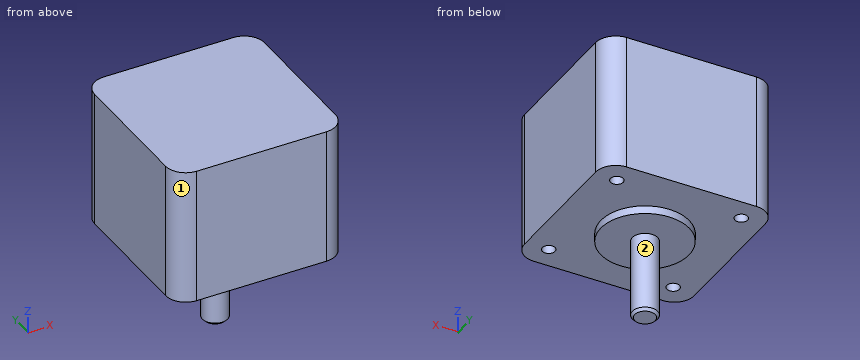
from build123d import *

# Parameters (mm, degrees)
SKETCH1_R           = 1.5875
BOSS_EXTRUDE1_DEPTH = 32
BOSS_EXTRUDE2_DEPTH = 2
SKETCH3_R           = 11
BOSS_EXTRUDE3_DEPTH = 2
SKETCH4_R           = 3.175
BOSS_EXTRUDE4_DEPTH = 20
CHAMFER1_SIZE       = 0.635


with BuildPart() as part:
    # Sketch1 → Boss-Extrude1 (new body)
    with BuildSketch(Plane.XY):
        with BuildLine():
            Line((-16.15, -21.15), (16.15, -21.15))
            ThreePointArc((16.15, -21.15), (19.685533906, -19.685533906), (21.15, -16.15))
            Line((21.15, -16.15), (21.15, 16.15))
            ThreePointArc((21.15, 16.15), (19.685533906, 19.685533906), (16.15, 21.15))
            Line((16.15, 21.15), (-16.15, 21.15))
            ThreePointArc((-16.15, 21.15), (-19.685533906, 19.685533906), (-21.15, 16.15))
            Line((-21.15, 16.15), (-21.15, -16.15))
            ThreePointArc((-21.15, -16.15), (-19.685533906, -19.685533906), (-16.15, -21.15))
        make_face()
        with Locations((15.5, 15.5)):
            Circle(SKETCH1_R, mode=Mode.SUBTRACT)
        with Locations((-15.5, 15.5)):
            Circle(SKETCH1_R, mode=Mode.SUBTRACT)
        with Locations((15.5, -15.5)):
            Circle(SKETCH1_R, mode=Mode.SUBTRACT)
        with Locations((-15.5, -15.5)):
            Circle(SKETCH1_R, mode=Mode.SUBTRACT)
    extrude(amount=BOSS_EXTRUDE1_DEPTH)

    # Sketch2 → Boss-Extrude2 (add)
    with BuildSketch(Plane.XY.offset(32)):
        with BuildLine():
            Line((-16.15, -21.15), (16.15, -21.15))
            ThreePointArc((16.15, -21.15), (19.685533906, -19.685533906), (21.15, -16.15))
            Line((21.15, -16.15), (21.15, 16.15))
            ThreePointArc((21.15, 16.15), (19.685533906, 19.685533906), (16.15, 21.15))
            Line((16.15, 21.15), (-16.15, 21.15))
            ThreePointArc((-16.15, 21.15), (-19.685533906, 19.685533906), (-21.15, 16.15))
            Line((-21.15, 16.15), (-21.15, -16.15))
            ThreePointArc((-21.15, -16.15), (-19.685533906, -19.685533906), (-16.15, -21.15))
        make_face()
    extrude(amount=BOSS_EXTRUDE2_DEPTH)

    # Sketch3 → Boss-Extrude3 (add)
    with BuildSketch(Plane(origin=(0, 0, 0), x_dir=(-1, 0, 0), z_dir=(0, 0, -1))):
        Circle(SKETCH3_R)
    extrude(amount=BOSS_EXTRUDE3_DEPTH)

    # Sketch4 → Boss-Extrude4 (add)
    with BuildSketch(Plane(origin=(0, 0, -2), x_dir=(-1, 0, 0), z_dir=(0, 0, -1))):
        Circle(SKETCH4_R)
    extrude(amount=BOSS_EXTRUDE4_DEPTH)

    # Chamfer1
    chamfer1_edges = [part.edges().sort_by_distance(p)[0] for p in [
        (3.175, 0, -22),
    ]]
    chamfer(chamfer1_edges, length=CHAMFER1_SIZE)


solid = part.part
Design review of the part built by this model. Coordinates are the model's own, in mm. Face numbers are marked on the shaded views. A direction names the side the tool comes from. Coordinates: 2 decimals unless noted, no trailing zeros. Order: outer loops, then holes, each group sorted by start corner. A loop starts at its lowest first (then second) coordinate and runs counter-clockwise, first axis right, second up.
Item 1: For the marked faces 1 and 2, list the 3-axis set-ups (+Z, -Z, +X, -X, +Y, -Y) from which the entire face can be reached by the end or side of a thin tool; tool diameter is ignored.
Item 2: Take a section at B-B, the plane x = 0. Write out the cut boundary in (y, z) (3 decimals).
Item 3: For line 1 (Y direction, x = -15.5, z = 18.5); line 2 (Y direction, x = 16, z = 28), list the stretches that pass through material, from the lowest coordinate up.
Item 4: For pin 1 Ø3 at (x, y) = (-3, 3) entering from -Z; pin 2 Ø5 at (x, y) = (7, 9) entering from -Z; pin 3 Ø3.5 at (x, y) = (-15.5, 16) entering from -Z, all flat-tipped, find the tip position at first contact; note any pin that passes through.
Item 5: Take a section at D-D, the plane x = 5. Write out the cut boundary in (y, z), then the cut area to 3 significant figures.
Item 6: Take a section at A-A, the plane z = 17. Count the separate pieces of the cut face and the enclosed holes in it, then the cut area to 3 significant figures.
Item 7: Take a section at C-C, the plane z = -4. Write out the cut boundary in (x, y) (3 decimals).
The answers:
1. face 1: +Z, -Z, -X, -Y
1. face 2: -Z
2. outline: (-21.15, 0) - (-11, 0) - (-11, -2) - (-3.175, -2) - (-3.175, -21.365) - (-2.54, -22) - (2.54, -22) - (3.175, -21.365) - (3.175, -2) - (11, -2) - (11, 0) - (21.15, 0) - (21.15, 34) - (-21.15, 34) - close
3. line 1: y = -21.15 to -17.09, -13.91 to 13.91, 17.09 to 21.15
3. line 2: y = -21.15 to -17.01, -13.99 to 13.99, 17.01 to 21.15
4. pin 1: stops at z = -21.8
4. pin 2: stops at z = -2
4. pin 3: stops at z = 0
5. outline: (-21.15, 0) - (-9.8, 0) - (-9.8, -2) - (9.8, -2) - (9.8, 0) - (21.15, 0) - (21.15, 34) - (-21.15, 34) - close
5. area: 1,480 mm2
6. separate pieces: 1
6. enclosed holes: 4
6. area: 1,740 mm2
7. outline: circle Ø6.35 at (0, 0)
